Can you work these out from the model? Positions are in its coordinate system, mm. Face numbers are marked on the shaded views. A direction names the side the tool comes from. Coordinates: 2 decimals unless noted, no trailing zeros. Order: outer loops, then holes, each group sorted by start corner. A loop starts at its lowest first (then second) coordinate and runs counter-clockwise, first axis right, second up. Notation, with made-up numbers: (37.5, 63) -> (83.5, 63) arc R28 ccw to (83.5, 93) -> close; hole circle Ø10 at (-23.75, 55). An arc over 180 degrees is marked (long way). Write item = value, one per line.
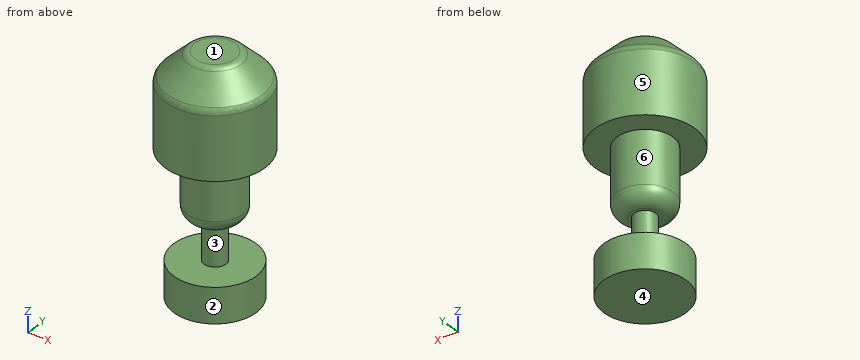
```python
from build123d import *

# Parameters (mm, degrees)
F0_R      = 28.5
F1_DEPTH  = 26.5
F2_R      = 16
F3_DEPTH  = 38
F4_R      = 8
F5_SIZE   = 15
F6_R      = 5
F7_R      = 6.25
F8_DEPTH  = 23
F9_R      = 23.5
F10_DEPTH = 20


with BuildPart() as f1:
    # F0 (on Top) → F1 (new body, symmetric)
    with BuildSketch(Plane.XY):
        Circle(F0_R)
    extrude(amount=F1_DEPTH, both=True)

    # F2 (on face) → F3 (join)
    with BuildSketch(Plane(origin=(0, 0, -26.5), x_dir=(1, 0, 0), z_dir=(0, 0, -1))):
        Circle(F2_R)
    extrude(amount=F3_DEPTH)

    # F4
    f4_edges = [f1.edges().sort_by_distance(p)[0] for p in [
        (-16, 0, -64.5),
    ]]
    fillet(f4_edges, radius=F4_R)

    # F5
    f5_edges = [f1.edges().sort_by_distance(p)[0] for p in [
        (-28.5, 0, 26.5),
    ]]
    chamfer(f5_edges, length=F5_SIZE)

    # F6
    f6_edges = [f1.edges().sort_by_distance(p)[0] for p in [
        (-28.5, 0, 11.5),
        (-13.5, 0, 26.5),
    ]]
    fillet(f6_edges, radius=F6_R)

    # F7 (on face) → F8 (join)
    with BuildSketch(Plane(origin=(0, 0, -64.5), x_dir=(1, 0, 0), z_dir=(0, 0, -1))):
        Circle(F7_R)
    extrude(amount=F8_DEPTH)

    # F9 (on face) → F10 (join)
    with BuildSketch(Plane(origin=(0, 0, -87.5), x_dir=(1, 0, 0), z_dir=(0, 0, -1))):
        Circle(F9_R)
    extrude(amount=F10_DEPTH)


solid = f1.part
```
Item 1: If we mould it in two halves opening along Z, with no side actions, what happens to the marked faces 1, 2, 3 and 4? For each: pulls with the +Z half, pulls with the -Z half, needs draft (parallel to the pull), parting line crosses it, or undercut.
A:
face_1 = pulls with the +Z half
face_2 = needs draft
face_3 = undercut
face_4 = pulls with the -Z half
Item 2: For the marked faces 5 and 6, which set-ups out of +Z, -Z, +X, -X, +Y, -Y let a thin tool reach every point of the face, with its end or its side?
A:
face_5 = +Z, -Z
face_6 = none
Item 3: I want a section at B-B, the plane z = -89.5. Please give me the cut outline in (x, y), plus the area to 3 significant figures.
A:
outline = circle Ø47 at (0, 0)
area = 1,730 mm2
Item 4: I'm going to push flat-ended pins straight in: P1, Ø2, axis at y = -14, z = -58.5, coming from the -X side (3 decimals); P2, Ø10, axis at y = 8, z = -89.5, coming from the +X side; P3, Ø4, axis at x = -21, y = -15, coming from the -Z side. Where does each tip first touch, or does it pass through?
A:
P1 = -8.945
P2 = 23.31
P3 = -26.5
Item 5: If I drill on probe 1 along Z at (x, y) = (-7, -2); probe 2 along Z at (x, y) = (-4, -10); probe 3 along X at (y, z) = (-9, -15), over which ranges is the centre line in solid material (lowest first)?
A:
probe_1 = -107.5 to -87.5, -64.5 to 26.5
probe_2 = -107.5 to -87.5, -64.01 to 26.5
probe_3 = -27.04 to 27.04
Item 6: I want a section at A-A, the plane z = -32. Please give me the cut outline in (x, y).
A:
outline = circle Ø32 at (0, 0)
